```python
from build123d import *

# Parameters (mm, degrees)
SKETCH1_R           = 25.1
SKETCH1_R_2         = 43.202132663
SKETCH1_R_3         = 7
SKETCH1_R_4         = 3.800397256
SKETCH1_R_5         = 2.770442617
SKETCH1_R_6         = 3.592040897
SKETCH1_R_7         = 3.686204525
SKETCH1_R_8         = 3.29684687
SKETCH1_R_9         = 3.69392349
SKETCH1_R_10        = 3.414332156
SKETCH1_R_11        = 3.736354481
SKETCH1_R_12        = 4.159658534
SKETCH1_R_13        = 3.983387515
SKETCH1_R_14        = 3.611599691
BOSS_EXTRUDE1_DEPTH = 30


with BuildPart() as part:
    # Sketch1 → Boss-Extrude1 (new body)
    with BuildSketch(Plane.XY):
        with BuildLine():
            Line((22.5, 72.746158915), (22.5, 0))
            Line((22.5, 0), (296.37, 0))
            Line((296.37, 0), (296.37, 183.19))
            ThreePointArc((296.37, 183.19), (230.582473324, 223.969990415), (204.87, 296.97598332))
            Line((204.87, 296.97598332), (204.87, 336.464053823))
            ThreePointArc((204.87, 336.464053823), (201.941067812, 343.535121635), (194.87, 346.464053823))
            Line((194.87, 346.464053823), (124, 346.464053823))
            ThreePointArc((124, 346.464053823), (116.928932188, 343.535121635), (114, 336.464053823))
            Line((114, 336.464053823), (114, 269.897959103))
            ThreePointArc((114, 269.897959103), (80.757131827, 188.408696007), (0, 153.424786226))
            ThreePointArc((0, 153.424786226), (-80.757131827, 188.408696007), (-114, 269.897959103))
            Line((-114, 269.897959103), (-114, 336.464053823))
            ThreePointArc((-114, 336.464053823), (-116.928932188, 343.535121635), (-124, 346.464053823))
            Line((-124, 346.464053823), (-194.87, 346.464053823))
            ThreePointArc((-194.87, 346.464053823), (-201.941067812, 343.535121635), (-204.87, 336.464053823))
            Line((-204.87, 336.464053823), (-204.87, 296.97598332))
            ThreePointArc((-204.87, 296.97598332), (-321.37, 180.47598332), (-437.87, 296.97598332))
            Line((-437.87, 296.97598332), (-437.87, 336.464053823))
            ThreePointArc((-437.87, 336.464053823), (-440.798932188, 343.535121635), (-447.87, 346.464053823))
            Line((-447.87, 346.464053823), (-494.813243917, 346.464053823))
            ThreePointArc((-494.813243917, 346.464053823), (-501.884311728, 343.535121635), (-504.813243917, 336.464053823))
            Line((-504.813243917, 336.464053823), (-504.813243917, 288.967719833))
            ThreePointArc((-504.813243917, 288.967719833), (-475.587111443, 184.338156739), (-396.37, 110))
            Line((-396.37, 110), (-318.87, 110))
            ThreePointArc((-318.87, 110), (-302.960097423, 103.409902577), (-296.37, 87.5))
            Line((-296.37, 87.5), (-296.37, 0))
            Line((-296.37, 0), (-22.5, 0))
            Line((-22.5, 0), (-22.5, 72.740041961))
            ThreePointArc((-22.5, 72.740041961), (-15.910273536, 88.652107355), (0, 95.246158915))
            ThreePointArc((0, 95.246158915), (15.909902577, 88.656061492), (22.5, 72.746158915))
        make_face()
        with Locations((-159.43, 91.5)):
            Circle(SKETCH1_R, mode=Mode.SUBTRACT)
        with Locations((-159.44, 161.5)):
            Circle(SKETCH1_R, mode=Mode.SUBTRACT)
        with Locations((159.44, 71.5)):
            Circle(SKETCH1_R, mode=Mode.SUBTRACT)
        with Locations((156.422663426, 141.434938908)):
            Circle(SKETCH1_R_2, mode=Mode.SUBTRACT)
        with Locations((-464.813243917, 207.5)):
            Circle(SKETCH1_R_3, mode=Mode.SUBTRACT)
        with Locations((-495.795209239, 273.49)):
            Circle(SKETCH1_R_4, mode=Mode.SUBTRACT)
        with Locations((-470.58146842, 280.390080126)):
            Circle(SKETCH1_R_5, mode=Mode.SUBTRACT)
        with Locations((-447.87, 273.49)):
            Circle(SKETCH1_R_6, mode=Mode.SUBTRACT)
        with Locations((-470.58146842, 315.390080126)):
            Circle(SKETCH1_R_7, mode=Mode.SUBTRACT)
        with Locations((-494.434659893, 328.473169293)):
            Circle(SKETCH1_R_8, mode=Mode.SUBTRACT)
        with Locations((-454.434659893, 328.473169293)):
            Circle(SKETCH1_R_9, mode=Mode.SUBTRACT)
        with Locations((-188.708856361, 288.967719833)):
            Circle(SKETCH1_R_10, mode=Mode.SUBTRACT)
        with Locations((-159.44, 296.97598332)):
            Circle(SKETCH1_R_11, mode=Mode.SUBTRACT)
        with Locations((-128.95804363, 288.967719833)):
            Circle(SKETCH1_R_12, mode=Mode.SUBTRACT)
        with Locations((-188.708856361, 332.039656125)):
            Circle(SKETCH1_R_13, mode=Mode.SUBTRACT)
        with Locations((-159.44, 331.97598332)):
            Circle(SKETCH1_R_10, mode=Mode.SUBTRACT)
        with Locations((-128.708856361, 332.039656125)):
            Circle(SKETCH1_R_14, mode=Mode.SUBTRACT)
        with Locations((159.434406699, 211.370118913)):
            Circle(SKETCH1_R, mode=Mode.SUBTRACT)
        with Locations((128.95804363, 288.967719833)):
            Circle(SKETCH1_R_12, mode=Mode.SUBTRACT)
        with Locations((188.708856361, 288.967719833)):
            Circle(SKETCH1_R_10, mode=Mode.SUBTRACT)
        with Locations((159.44, 296.97598332)):
            Circle(SKETCH1_R_11, mode=Mode.SUBTRACT)
        with Locations((128.708856361, 332.039656125)):
            Circle(SKETCH1_R_14, mode=Mode.SUBTRACT)
        with Locations((159.44, 331.97598332)):
            Circle(SKETCH1_R_10, mode=Mode.SUBTRACT)
        with Locations((188.708856361, 332.039656125)):
            Circle(SKETCH1_R_13, mode=Mode.SUBTRACT)
    extrude(amount=BOSS_EXTRUDE1_DEPTH)


solid = part.part
```
Geometry: final body of the model. Coordinates: model frame, mm. A direction names the side the tool comes from. Give positions to 0.01 mm unless a question says otherwise; leave off trailing zeros. Order: outer loops, then holes, each group sorted by start corner. A loop starts at its lowest first (then second) coordinate and runs counter-clockwise, first axis right, second up. Notation, with made-up numbers: M -5.75,1 L 9.25,1 A30 cw 9.25,30 Z; hole C 51,3 d6. An arc over 180 degrees is marked long. Answer as CSV lines item,"result". Start each with the question number.
1) Cut plane D-D (z = 21). State how many separate pieces and enclosed holes the cut face has, then the cut area to 3 significant figures.
2) First-contact query: P1, Ø15, axis at y = 21.5, z = 15.5, coming from the -X side; P2, Ø1, axis at x = -217, z = 19.5, coming from the +Y side; P3, Ø4, axis at x = 60.5, z = 9, coming from the +Y side. Flat tips, straight axial feed; report the tip coordinate or a pass-through.
3) Line query: line 1 (Y direction, x = 159.44, z = 23.5); line 2 (X direction, y = 31, z = 5); line 3 (X direction, y = 307, z = 17.5). Output: solid intervals per line, ascending. Write a range as from..to.
4) Mould query, pull axis Y, two halves, no side actions, for faces 1 (the cylindrical face through (-476.38, 185.66, 14.79)), 2 (the cylindrical face through (81.64, 189.32, 14.79)), 3 (the cylindrical face through (-179.35, 76.23, 14.79)). Classes: +Y half, -Y half, draft (parallel to the pull), parting line (faces both ways), or undercut.
5) Cut plane B-B (y = 247). Output: boundary loops of the cut face in (x, z).
6) Cut plane C-C (x = -330). Output: boundary loops of the cut face in (y, z), then the cut area to 3 significant figures.
7) Cut plane A-A (y = 161.5). Output: boundary loops of the cut face in (x, z), then the cut area to 3 significant figures.
8) Set-up query: faces 4 (the cylindrical face through (-79.87, 187.51, 14.79)), 5 (the flat face through (-22.5, 36, 15)), 6 (the flat face through (-159, 346.464, 15)). Return all of +Z, -Z, +X, -X, +Y, -Y with unobstructed straight access to the full face (end or side cutting, diameter ignored); none if empty.
Findings below:
1,separate pieces,"1"
1,enclosed holes,"24"
1,area,"147,000 mm²"
2,P1,"stops at x = -296.37"
2,P2,"stops at y = 246.24"
2,P3,"stops at y = 173.22"
3,line 1,"y = 0..46.4, 96.6..98.34, 184.53..186.27, 236.47..293.24, 300.71..328.56, 335.39..346.46"
3,line 2,"x = -296.37..-22.5, 22.5..296.37"
3,line 3,"x = -504.81..-437.87, -204.87..-114, 114..204.87"
4,face 1,"-Y half"
4,face 2,"+Y half"
4,face 3,"undercut"
5,outline,"M -500.4,0 L -426.61,0 L -426.61,30 L -500.4,30 Z; M -216.13,0 L -111.73,0 L -111.73,30 L -216.13,30 Z; M 111.73,0 L 216.13,0 L 216.13,30 L 111.73,30 Z"
6,outline,"M 110,0 L 180.8,0 L 180.8,30 L 110,30 Z"
6,area,"2,120 mm²"
7,outline,"M -459.49,0 L -184.54,0 L -184.54,30 L -459.49,30 Z; M -134.34,0 L -40.19,0 L -40.19,30 L -134.34,30 Z; M 40.19,0 L 118.16,0 L 118.16,30 L 40.19,30 Z; M 194.68,0 L 296.37,0 L 296.37,30 L 194.68,30 Z"
7,area,"16,500 mm²"
8,face 4,"+Z, -Z, +Y"
8,face 5,"+Z, -Z, -Y"
8,face 6,"+Z, -Z, +X, -X, +Y"
